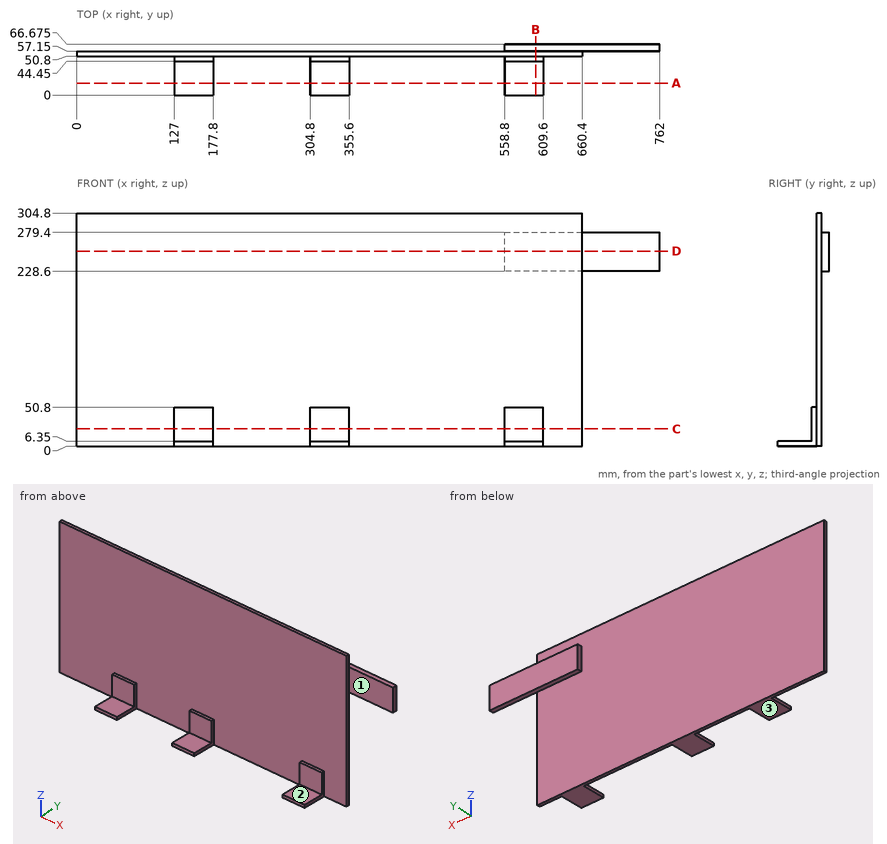
Job drawing, mm, ordinate dimensions from the low corner. One solid piece. A direction names the side the tool comes from. Give positions to 0.01 mm unless a question says otherwise; leave off trailing zeros. Loops run counter-clockwise (first coordinate to the right, second up) from the corner with the lowest first, then second, coordinate; pieces in that order, holes last. Notation, with made-up numbers: (-27.5, 14) -> (-9.5, 14) arc R24 cw to (-9.5, 34) -> close; hole circle Ø4 at (82, 61.25). An arc over 180 degrees is marked (long way). Write each question's results on one line, items separated by ' | '.
(1) Probe line 1 along Y through (x, z) = (72, 59.5); line 2 along Z through (x, y) = (588.5, 20.5); line 3 along X through (y, z) = (52, 248). List the from-to ranges inside material, lowest first.
Geometry results:
line 1: y = 50.8 to 57.15 | line 2: z = 0 to 6.35 | line 3: x = 0 to 660.4
(2) Tool access for the marked faces 1, 2 and 3: list every direction of +Z, -Z, +X, -X, +Y, -Y with a clear straight run to the whole face (end or side of a thin tool).
Geometry results:
face 1: +Z, -Z, +X, -Y | face 2: +Z, +X, -X, -Y | face 3: -Z, +X, -X, +Y, -Y
(3) Cut at A-A on y = 15.5. List the corners of the cut face in (x, z).
Geometry results:
outline: (127, 0) -> (177.8, 0) -> (177.8, 6.35) -> (127, 6.35) -> close; (304.8, 0) -> (355.6, 0) -> (355.6, 6.35) -> (304.8, 6.35) -> close; (558.8, 0) -> (609.6, 0) -> (609.6, 6.35) -> (558.8, 6.35) -> close
(4) Cut at B-B on x = 599.5. List the corners of the cut face in (y, z) (3 decimals).
Geometry results:
outline: (0, 0) -> (57.15, 0) -> (57.15, 228.6) -> (66.675, 228.6) -> (66.675, 279.4) -> (57.15, 279.4) -> (57.15, 304.8) -> (50.8, 304.8) -> (50.8, 50.8) -> (44.45, 50.8) -> (44.45, 6.35) -> (0, 6.35) -> close
(5) Cut at D-D on z = 255. List the corners of the cut face in (x, y) (3 decimals), and give its area (3 significant figures).
Geometry results:
outline: (0, 50.8) -> (660.4, 50.8) -> (660.4, 57.15) -> (762, 57.15) -> (762, 66.675) -> (558.8, 66.675) -> (558.8, 57.15) -> (0, 57.15) -> close | area: 6,130 mm²
(6) Flat gauge pins, fed straight in: pin 1 Ø12 at (x, z) = (128, 224.5) entering from +Y; pin 2 Ø6 at (y, z) = (46, 204) entering from +X; pin 3 Ø3 at (x, y) = (656, 62.5) entering from -Z; pin 4 Ø22 at (x, z) = (586, 39.5) entering from -Y. Where does each tip first touch, or does it go through?
Geometry results:
pin 1: stops at y = 57.15 | pin 2: passes through | pin 3: stops at z = 228.6 | pin 4: stops at y = 44.45
(7) Cut at C-C on z = 22.5. List the corners of the cut face in (x, y), and give its area (3 significant figures).
Geometry results:
outline: (0, 50.8) -> (127, 50.8) -> (127, 44.45) -> (177.8, 44.45) -> (177.8, 50.8) -> (304.8, 50.8) -> (304.8, 44.45) -> (355.6, 44.45) -> (355.6, 50.8) -> (558.8, 50.8) -> (558.8, 44.45) -> (609.6, 44.45) -> (609.6, 50.8) -> (660.4, 50.8) -> (660.4, 57.15) -> (0, 57.15) -> close | area: 5,160 mm²
